Can you work these out from the model? Positions are in its coordinate system, mm. A direction names the side the tool comes from. Round coordinates to 2 decimals unless told otherwise and drop trailing zeros. Loops run counter-clockwise (first coordinate to the right, second up) from the corner with the lowest first, then second, coordinate; pieces in that order, holes last. Notation, with made-up numbers: (26.25, 84) - (48.25, 84) arc R27 ccw to (48.25, 122) - close; hole circle Ø4 at (61.5, 3). An arc over 180 degrees is marked (long way). Answer as CSV lines item,"result".
```python
from build123d import *

# Parameters (mm, degrees)
SKETCH1_W           = 50
SKETCH1_H           = 36
SKETCH1_R           = 1.55
BOSS_EXTRUDE1_DEPTH = 1.6
SKETCH2_W           = 5.5
SKETCH2_H           = 30
BOSS_EXTRUDE2_DEPTH = 1.5


with BuildPart() as part:
    # Sketch1 → Boss-Extrude1 (new body)
    with BuildSketch(Plane(origin=(0, 0, 0), x_dir=(1, 0, 0), z_dir=(0, 1, 0))):
        Rectangle(SKETCH1_W, SKETCH1_H)
        with Locations(Location((-15.5, 15, 0), (0, 0, 270))):
            Circle(SKETCH1_R, mode=Mode.SUBTRACT)
        with Locations(Location((-15.5, -15, 0), (0, 0, 90))):
            Circle(SKETCH1_R, mode=Mode.SUBTRACT)
        with Locations(Location((14.5, 15, 0), (0, 0, 270))):
            Circle(SKETCH1_R, mode=Mode.SUBTRACT)
        with Locations(Location((14.5, -15, 0), (0, 0, 90))):
            Circle(SKETCH1_R, mode=Mode.SUBTRACT)
    extrude(amount=BOSS_EXTRUDE1_DEPTH)

    # Sketch2 → Boss-Extrude2 (add)
    with BuildSketch(Plane(origin=(0, 1.6, 0), x_dir=(1, 0, 0), z_dir=(0, 1, 0))):
        with Locations((20.45, 0)):
            Rectangle(SKETCH2_W, SKETCH2_H)
    extrude(amount=BOSS_EXTRUDE2_DEPTH)


solid = part.part
```
Q1. Imagine slicing it at B-B (y = 0.65). Write out the boundary of the cut face in (x, z), then the cut area to 3 significant figures.
Checks:
outline,"(-25, -18) - (25, -18) - (25, 18) - (-25, 18) - close; hole circle Ø3.1 at (-15.5, -15); hole circle Ø3.1 at (-15.5, 15); hole circle Ø3.1 at (14.5, -15); hole circle Ø3.1 at (14.5, 15)"
area,"1,770 mm²"
Q2. On a 3-axis mill with a long thin cutter (end or side, diameter ignored), from which of +Z, -Z, +X, -X, +Y, -Y can I reach the whole of each face in a straight line? I mean faces 1 (the flat face through (20, 2, -15)), 2 (the flat face through (17.7, 2, 0)), 3 (the flat face through (20, 2, 15)), 4 (the flat face through (0, 0, 0)). Say none if no direction works.
Checks:
face 1,"-Z, +X, -X, +Y"
face 2,"+Z, -Z, -X, +Y"
face 3,"+Z, +X, -X, +Y"
face 4,"+Z, -Z, +X, -X, -Y"
Q3. Imagine slicing it at C-C (x = 20). Write out the boundary of the cut face in (y, z), then the cut area to 3 significant figures.
Checks:
outline,"(0, -18) - (1.6, -18) - (1.6, -15) - (3.1, -15) - (3.1, 15) - (1.6, 15) - (1.6, 18) - (0, 18) - close"
area,"103 mm²"
Q4. If I drill on line 1 along X through (y, z) = (0.5, 15); line 2 along X through (y, z) = (1.75, 8); line 3 along Y through (x, z) = (-13, 8.5), over which ranges is the centre line in solid material (lowest first)? Write a range as [from, to].
Checks:
line 1,"[-25, -17.05], [-13.95, 12.95], [16.05, 25]"
line 2,"[17.7, 23.2]"
line 3,"[0, 1.6]"
Q5. Imagine slicing it at D-D (z = 10). Write out the boundary of the cut face in (x, y).
Checks:
outline,"(-25, 0) - (25, 0) - (25, 1.6) - (23.2, 1.6) - (23.2, 3.1) - (17.7, 3.1) - (17.7, 1.6) - (-25, 1.6) - close"
Q6. We'd pull the mould along X, two halves only. Please class faces 5 (the flat face through (0, 1, -18)), 6 (the cylindrical face through (13.45, 0.79, 16.14)), 7 (the flat face through (23.2, 2, 0)): pulls with the +X half, pulls with the -X half, needs draft (parallel to the pull), parting line crosses it, or undercut.
Checks:
face 5,"needs draft"
face 6,"undercut"
face 7,"pulls with the +X half"
Q7. Imagine slicing it at A-A (x = 14.5). Write out the boundary of the cut face in (y, z), then the cut area to 3 significant figures.
Checks:
outline,"(0, -18) - (1.6, -18) - (1.6, -16.55) - (0, -16.55) - close; (0, -13.45) - (1.6, -13.45) - (1.6, 13.45) - (0, 13.45) - close; (0, 16.55) - (1.6, 16.55) - (1.6, 18) - (0, 18) - close"
area,"47.7 mm²"
Q8. I'm going to push flat-ended pins straight in: pin 1 Ø1.5 at (y, z) = (2.5, -5) entering from +X; pin 2 Ø11 at (x, z) = (-8, 6.5) entering from +Y; pin 3 Ø0.8 at (y, z) = (2.5, -1.5) entering from -X; pin 4 Ø2.5 at (x, z) = (-15.5, 15) entering from -Y. Where does each tip first touch, or does it pass through?
Checks:
pin 1,"x = 23.2"
pin 2,"y = 1.6"
pin 3,"x = 17.7"
pin 4,"through"
